```python
from build123d import *

# Parameters (mm, degrees)
SKETCH1_R           = 17.5
BOSS_EXTRUDE1_DEPTH = 57.1
SKETCH2_R           = 16
BOSS_EXTRUDE2_DEPTH = 11
SKETCH3_R           = 16
BOSS_EXTRUDE3_DEPTH = 41.9
SKETCH4_R           = 1.5
CUT_EXTRUDE2_DEPTH  = 15
BOSS_EXTRUDE5_DEPTH = 3.7
SKETCH7_R           = 3
BOSS_EXTRUDE6_DEPTH = 15.5
CUT_EXTRUDE3_DEPTH  = 10


with BuildPart() as part:
    # Sketch1 → Boss-Extrude1 (new body)
    with BuildSketch(Plane(origin=(0, 0, 0), x_dir=(1, 0, 0), z_dir=(0, 1, 0))):
        Circle(SKETCH1_R)
    extrude(amount=BOSS_EXTRUDE1_DEPTH)

    # Sketch2 → Boss-Extrude2 (add)
    with BuildSketch(Plane.XZ):
        Circle(SKETCH2_R)
    extrude(amount=BOSS_EXTRUDE2_DEPTH)

    # Sketch3 → Boss-Extrude3 (add)
    with BuildSketch(Plane(origin=(0, 57.1, 0), x_dir=(1, 0, 0), z_dir=(0, 1, 0))):
        Circle(SKETCH3_R)
    extrude(amount=BOSS_EXTRUDE3_DEPTH)

    # Sketch4 → Cut-Extrude2 (cut)
    with BuildSketch(Plane(origin=(0, 99, 0), x_dir=(1, 0, 0), z_dir=(0, 1, 0))):
        with Locations((12.012324504, 4.970317898)):
            Circle(SKETCH4_R)
        with Locations((-4.970317898, 12.012324504)):
            Circle(SKETCH4_R)
        with Locations((-12.012324504, -4.970317898)):
            Circle(SKETCH4_R)
        with Locations((4.970317898, -12.012324504)):
            Circle(SKETCH4_R)
    extrude(amount=-CUT_EXTRUDE2_DEPTH, mode=Mode.SUBTRACT)

    # Sketch6 → Boss-Extrude5 (add)
    with BuildSketch(Plane(origin=(0, 99, 0), x_dir=(1, 0, 0), z_dir=(0, 1, 0))):
        with BuildLine():
            Line((-9.983215116, -0.579151054), (-6.643996337, 7.473774995))
            ThreePointArc((-6.643996337, 7.473774995), (3.830346634, 9.237339696), (9.983215116, 0.579151054))
            Line((9.983215116, 0.579151054), (6.643996337, -7.473774995))
            ThreePointArc((6.643996337, -7.473774995), (-3.830346634, -9.237339696), (-9.983215116, -0.579151054))
        make_face()
    extrude(amount=BOSS_EXTRUDE5_DEPTH)

    # Sketch7 → Boss-Extrude6 (add)
    with BuildSketch(Plane(origin=(0, 102.7, 0), x_dir=(1, 0, 0), z_dir=(0, 1, 0))):
        Circle(SKETCH7_R)
    extrude(amount=BOSS_EXTRUDE6_DEPTH)

    # Sketch8 → Cut-Extrude3 (cut)
    with BuildSketch(Plane(origin=(0, 118.2, 0), x_dir=(1, 0, 0), z_dir=(0, 1, 0))):
        with BuildLine():
            Line((-1.883851207, 2.334760079), (2.334760079, 1.883851207))
            ThreePointArc((2.334760079, 1.883851207), (0.318840721, 2.983008648), (-1.883851207, 2.334760079))
        make_face()
    extrude(amount=-CUT_EXTRUDE3_DEPTH, mode=Mode.SUBTRACT)


solid = part.part
```
Input: part model. Units: mm. Frame: model coordinates. A direction names the side the tool comes from. Round coordinates to 2 decimals unless told otherwise and drop trailing zeros. Loops run counter-clockwise (first coordinate to the right, second up) from the corner with the lowest first, then second, coordinate; pieces in that order, holes last. Notation, with made-up numbers: (-22, 56) -> (-7, 56) arc R4 ccw to (-7, 61) -> close; hole circle Ø8 at (11.5, 60.25). An arc over 180 degrees is marked (long way). Write each question's results on one line, items separated by ' | '.
1. Section B-B (y = 67.5). Return loops of the section in (x, z), and give its area (3 significant figures).
Geometry results:
outline: circle Ø32 at (0, 0) | area: 804 mm2
2. Section D-D (y = 110.5). Return loops of the section in (x, z).
Geometry results:
outline: (-1.88, -2.33) -> (2.33, -1.88) arc R3 ccw (long way) to start
3. Set-up query: faces 4 (the face through (0.196, 113.27, -2.112)), 5 (the face through (-8.337, 100.824, -3.391)), 6 (the face through (5, 84, 12)). Return all of +Z, -Z, +X, -X, +Y, -Y with unobstructed straight access to the full face (end or side cutting, diameter ignored); none if empty.
Geometry results:
face 4: -Z, +X, +Y | face 5: -Z, -X, +Y | face 6: +Y
4. First-contact query: P1, Ø5, axis at x = -10.5, z = 3, coming from the +Y side; P2, Ø16, axis at x = -3, z = -3.5, coming from the +Y side; P3, Ø1, axis at x = -8.5, y = 37, coming from the -Z side; P4, Ø1, axis at x = -11, z = 10, coming from the +Y side. Flat tips, straight axial feed; report the tip coordinate or a pass-through.
Geometry results:
P1: y = 102.7 | P2: y = 118.2 | P3: z = -15.56 | P4: y = 99
5. Section A-A (x = 0). Return loops of the section in (y, z), and give its area (3 significant figures).
Geometry results:
outline: (-11, -16) -> (0, -16) -> (0, -17.5) -> (57.1, -17.5) -> (57.1, -16) -> (99, -16) -> (99, -10) -> (102.7, -10) -> (102.7, -3) -> (108.2, -3) -> (108.2, -2.13) -> (118.2, -2.13) -> (118.2, 3) -> (102.7, 3) -> (102.7, 10) -> (99, 10) -> (99, 16) -> (57.1, 16) -> (57.1, 17.5) -> (0, 17.5) -> (0, 16) -> (-11, 16) -> close | area: 3,850 mm2
6. Ray query, line 1 (X direction, y = 77, z = -12.5); line 2 (Y direction, x = 15, z = -6); line 3 (Y direction, x = 6, z = -4). Return the intervals inside material, ascending. Write a range as from..to.
Geometry results:
line 1: -9.99..9.99 | line 2: 0..57.1 | line 3: -11..102.7
7. Mould query, pull axis Z, two halves, no side actions, for faces 1 (the face through (-0.65, 110.34, 2.93)), 2 (the face through (7.7, 0, 14.2)), 3 (the face through (4.645, 91.605, 13.477)). Classes: +Z half, -Z half, draft (parallel to the pull), parting line (faces both ways), or undercut.
Geometry results:
face 1: parting line | face 2: draft | face 3: undercut
8. Section C-C (x = 8.5). Return loops of the section in (y, z).
Geometry results:
outline: (-11, -13.56) -> (0, -13.56) -> (0, -15.3) -> (57.1, -15.3) -> (57.1, -13.56) -> (99, -13.56) -> (99, -5.27) -> (102.7, -5.27) -> (102.7, 3) -> (99, 3) -> (99, 13.56) -> (57.1, 13.56) -> (57.1, 15.3) -> (0, 15.3) -> (0, 13.56) -> (-11, 13.56) -> close
